Read the model definition and answer for the solid it produces. Units are mm, in the model's axes. Give positions to 0.01 mm unless a question says otherwise; leave off trailing zeros. Write each loop counter-clockwise with the first axis right and the second up, starting at its lowest first coordinate (ties: lowest second). Pieces come first, ordered by that corner, then holes. Notation, with made-up numbers: (76.25, -8.75) - (88.25, -8.75) arc R22 ccw to (88.25, 15.25) - close; hole circle Ø11 at (-0.5, 75). An arc over 180 degrees is marked (long way). Use CSV: the item, a comma, the result in double quotes. Start each with the question number.
from build123d import *

# Parameters (mm, degrees)
SKETCH1_W           = 150
SKETCH1_H           = 83.6
BOSS_EXTRUDE1_DEPTH = 1
SKETCH2_W           = 54
SKETCH2_H           = 25
CUT_EXTRUDE1_DEPTH  = 86.867572459
SKETCH3_R           = 2.5
CUT_EXTRUDE2_DEPTH  = 6.5
CUT_EXTRUDE3_DEPTH  = 10
FILLET1_R           = 10
SKETCH5_W           = 150
SKETCH5_H           = 5
CUT_EXTRUDE4_DEPTH  = 10


with BuildPart() as part:
    # Sketch1 → Boss-Extrude1 (new body)
    with BuildSketch(Plane.XY):
        Rectangle(SKETCH1_W, SKETCH1_H)
    extrude(amount=BOSS_EXTRUDE1_DEPTH)

    # Sketch2 → Cut-Extrude1 (cut, through all)
    with BuildSketch(Plane.XY.offset(1)):
        with Locations((0, -6.3)):
            Rectangle(SKETCH2_W, SKETCH2_H)
    extrude(amount=-CUT_EXTRUDE1_DEPTH, mode=Mode.SUBTRACT)

    # Sketch3 → Cut-Extrude2 (cut)
    with BuildSketch(Plane.XY.offset(1)):
        with Locations((-70, 16.72)):
            Circle(SKETCH3_R)
        with Locations((-70, -13.28)):
            Circle(SKETCH3_R)
        with Locations((70, 16.72)):
            Circle(SKETCH3_R)
        with Locations((70, -13.28)):
            Circle(SKETCH3_R)
    extrude(amount=-CUT_EXTRUDE2_DEPTH, mode=Mode.SUBTRACT)

    # Sketch4 → Cut-Extrude3 (cut)
    with BuildSketch(Plane.XY.offset(1)):
        Polygon((0, 34.8), (12, 34.8), (12, 41.8), (-12, 41.8), (-12, 34.8), align=None)
    extrude(amount=-CUT_EXTRUDE3_DEPTH, mode=Mode.SUBTRACT)

    # Fillet1
    fillet1_edges = [part.edges().sort_by_distance(p)[0] for p in [
        (27, -18.8, 0.5),
        (-27, -18.8, 0.5),
        (-27, 6.2, 0.5),
        (27, 6.2, 0.5),
    ]]
    fillet(fillet1_edges, radius=FILLET1_R)

    # Sketch5 → Cut-Extrude4 (cut)
    with BuildSketch(Plane.XY.offset(1)):
        with Locations((0, -39.3)):
            Rectangle(SKETCH5_W, SKETCH5_H)
    extrude(amount=-CUT_EXTRUDE4_DEPTH, mode=Mode.SUBTRACT)


solid = part.part
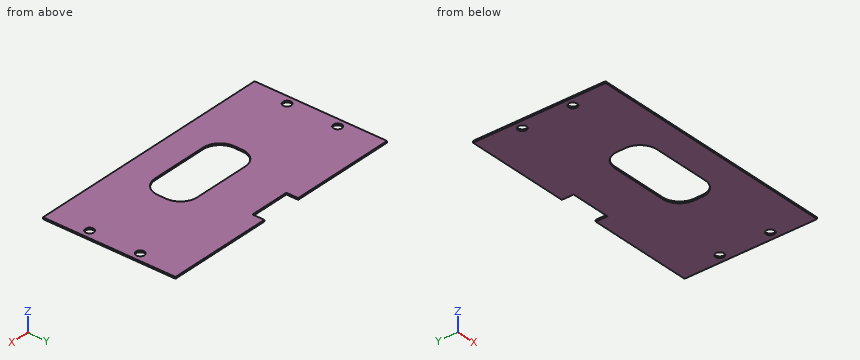
(1) The part is cut by section A-A on y = 37.5. Write down the section's boundary in (x, z).
(2) Consider probe 1 along Y at (x, z) = (70, 0.6); probe 2 along X at (y, z) = (36, 0.9); probe 3 along X at (y, z) = (-5, 0.65). Determine where each line is inside the solid, lowest interval first.
(3) Given P1, Ø0.5, axis at x = 4.5, z = 0.5, coming from the +Y side, flat-ended and moving along its own axis, determine where the tip first touches the part or whether it passes through.
(4) The part is cut by section B-B on x = 0.5. Write down the section's boundary in (y, z), plus the area to 3 significant figures.
(5) The part is cut by section C-C on z = 0.6. Write down the section's boundary in (x, y), plus the area to 3 significant figures.
(6) The part is cut by section D-D on y = 16.72. Write down the section's boundary in (x, z), plus the area to 3 significant figures.
Reported:
1,outline,"(-75, 0) - (-12, 0) - (-12, 1) - (-75, 1) - close; (12, 0) - (75, 0) - (75, 1) - (12, 1) - close"
2,probe 1,"-36.8 to -15.78, -10.78 to 14.22, 19.22 to 41.8"
2,probe 2,"-75 to -12, 12 to 75"
2,probe 3,"-75 to -27, 27 to 75"
3,P1,"y = 34.8"
4,outline,"(-36.8, 0) - (-18.8, 0) - (-18.8, 1) - (-36.8, 1) - close; (6.2, 0) - (34.8, 0) - (34.8, 1) - (6.2, 1) - close"
4,area,"46.6 mm²"
5,outline,"(-75, -36.8) - (75, -36.8) - (75, 41.8) - (12, 41.8) - (12, 34.8) - (-12, 34.8) - (-12, 41.8) - (-75, 41.8) - close; hole circle Ø5 at (-70, -13.28); hole circle Ø5 at (-70, 16.72); hole (-27, -8.8) arc R10 ccw to (-17, -18.8) - (17, -18.8) arc R10 ccw to (27, -8.8) - (27, -3.8) arc R10 ccw to (17, 6.2) - (-17, 6.2) arc R10 ccw to (-27, -3.8) - close; hole circle Ø5 at (70, -13.28); hole circle Ø5 at (70, 16.72)"
5,area,"10,300 mm²"
6,outline,"(-75, 0) - (-72.5, 0) - (-72.5, 1) - (-75, 1) - close; (-67.5, 0) - (67.5, 0) - (67.5, 1) - (-67.5, 1) - close; (72.5, 0) - (75, 0) - (75, 1) - (72.5, 1) - close"
6,area,"140 mm²"
